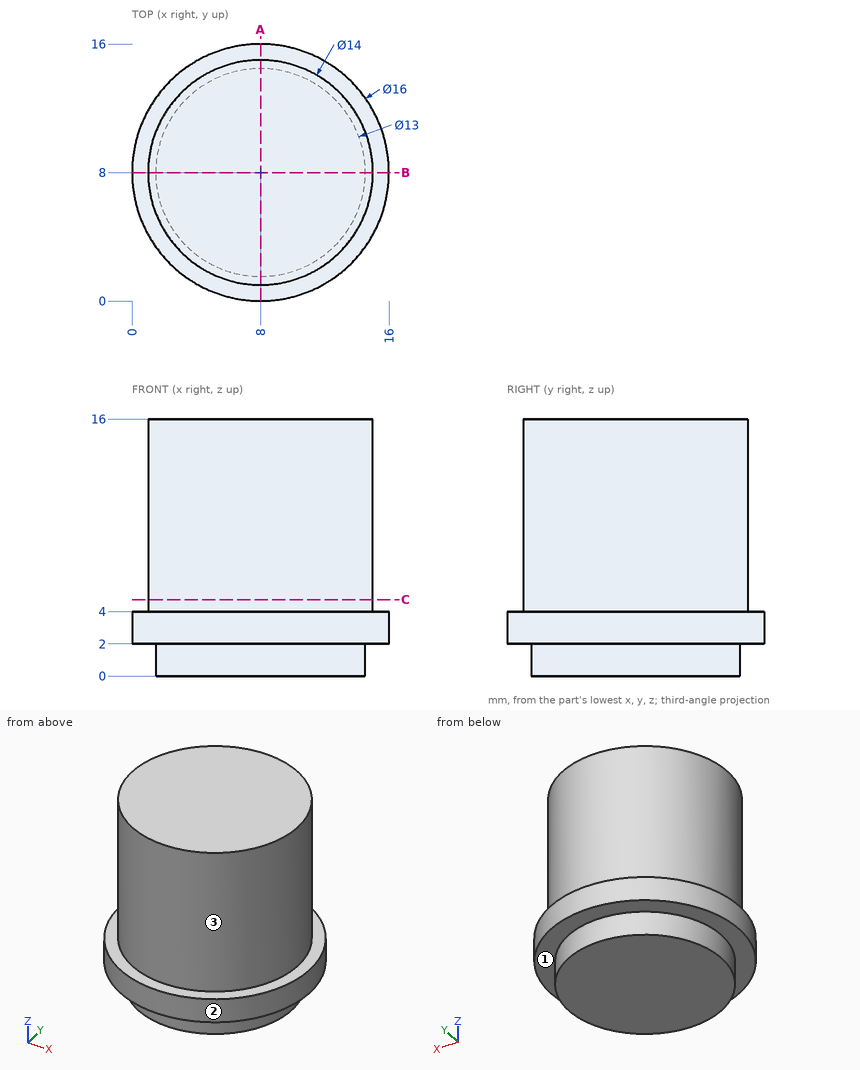
Part print with two shaded views. Sizes in mm from the minimum x, y, z corner. A direction names the side the tool comes from. Round coordinates to 2 decimals unless told otherwise and drop trailing zeros. Order: outer loops, then holes, each group sorted by start corner. A loop starts at its lowest first (then second) coordinate and runs counter-clockwise, first axis right, second up. Notation, with made-up numbers: M -15,48.5 L -10,48.5 A16 cw -10,78.5 Z; hole C -35,-13 d8. An arc over 180 degrees is marked long. Use CSV: the item, a comma, the result in double quotes.
Item 1: Saw through at A-A (x = 8). List the corners of the cut face in (y, z).
Worked answers:
outline,"M 0,2 L 1.5,2 L 1.5,0 L 14.5,0 L 14.5,2 L 16,2 L 16,4 L 15,4 L 15,16 L 1,16 L 1,4 L 0,4 Z"
Item 2: Saw through at C-C (z = 4.75). List the corners of the cut face in (x, y).
Worked answers:
outline,"C 8,8 d14"
Item 3: Which spindle directions (+Z, -Z, +X, -X, +Y, -Y) get a long thin tool onto all of the face, cutting with end or side? Do the marked faces 1, 2 and 3. Say none if no direction does.
Worked answers:
face 1,"-Z"
face 2,"+Z, -Z"
face 3,"+Z"
Item 4: Probe probe 1 along Z at (x, y) = (2.75, 13.5); probe 2 along Y at (x, z) = (8, 9.5); probe 3 along X at (y, z) = (4.5, 10.5). List the from-to ranges inside material, lowest first.
Worked answers:
probe 1,"2 to 4"
probe 2,"1 to 15"
probe 3,"1.94 to 14.06"
Item 5: Pin check, flat tips, straight feed: pin 1 (4 mm diameter, centred on y = 14, z = 4.5, fed in from -X); pin 2 (8 mm diameter, centred on x = 6.5, y = 10.5, fed in from -Z); pin 3 (8 mm diameter, centred on x = 8, z = 11.5, fed in from -Y); pin 4 (3 mm diameter, centred on x = 11, z = 10.5, fed in from -Y). Stop position of each tip, or through.
Worked answers:
pin 1,"x = 1.11"
pin 2,"z = 0"
pin 3,"y = 1"
pin 4,"y = 1.16"
